Source: CAD feature listing. Evaluate the final solid. Frame: model axes, mm. Give positions to 0.01 mm unless a question says otherwise; leave off trailing zeros. Loops run counter-clockwise (first coordinate to the right, second up) from the corner with the lowest first, then second, coordinate; pieces in that order, holes last. Notation, with made-up numbers: M 2.25,-37.75 L 36.25,-37.75 A21 cw 36.25,-14.75 Z; hole C 52.5,36 d10. An arc over 180 degrees is marked long. Write item = value, one per line.
from build123d import *

# Parameters (mm, degrees)
SKETCH1_4_R         = 3
SKETCH1_4_W         = 5.2
SKETCH1_4_H         = 20.6
BOSS_EXTRUDE2_DEPTH = 4
SKETCH1_5_R         = 3
SKETCH1_5_R_2       = 1
BOSS_EXTRUDE3_DEPTH = 2


with BuildPart() as part:
    # Sketch1_4 → Boss-Extrude2 (new body)
    with BuildSketch(Plane(origin=(0, 0, 0), x_dir=(1, 0, 0), z_dir=(0, 1, 0))):
        Polygon((-61.058774723, -67.225766481), (-46.058774723, -67.225766481), (-46.058774723, -57.925766481), (-16.058774723, -57.925766481), (-16.058774723, -47.925766481), (-46.058065355, -47.925766481), (-46.058065355, -38.625766481), (-46.058774723, 52.774233519), (-46.058774723, 62.074233519), (-16.058774723, 62.074233519), (-16.058774723, 72.074233519), (-46.058065355, 72.074233519), (-46.058065355, 81.374233519), (-61.058065355, 81.374233519), (-61.058065355, 72.074233519), (-111.058065355, 72.074233519), (-111.058065355, 62.074233519), (-61.058774723, 62.074233519), (-61.058774723, 52.774233519), (-61.058065355, -38.625766481), (-61.058065355, -47.925766481), (-111.058065355, -47.925766481), (-111.058065355, -57.925766481), (-61.058774723, -57.925766481), align=None)
        with Locations((-96.731187499, 67.074233519)):
            Circle(SKETCH1_4_R, mode=Mode.SUBTRACT)
        with Locations((-23.608327945, 67.074233519)):
            Circle(SKETCH1_4_R, mode=Mode.SUBTRACT)
        with Locations((-96.731187499, -52.925766481)):
            Circle(SKETCH1_4_R, mode=Mode.SUBTRACT)
        with Locations((-23.608327945, -52.925766481)):
            Circle(SKETCH1_4_R, mode=Mode.SUBTRACT)
        with Locations((-53.558065355, -52.925766481)):
            Rectangle(SKETCH1_4_W, SKETCH1_4_H, mode=Mode.SUBTRACT)
        with Locations((-53.558065355, 67.074233519)):
            Rectangle(SKETCH1_4_W, SKETCH1_4_H, mode=Mode.SUBTRACT)
    extrude(amount=BOSS_EXTRUDE2_DEPTH)

    # Sketch1_5 → Boss-Extrude3 (add)
    with BuildSketch(Plane(origin=(0, 0, 0), x_dir=(1, 0, 0), z_dir=(0, 1, 0))):
        Polygon((-61.058774723, -57.925766481), (-61.058774723, -67.225766481), (-46.058774723, -67.225766481), (-46.058774723, -57.925766481), (-16.058774723, -57.925766481), (-16.058774723, -47.925766481), (-46.058065355, -47.925766481), (-46.058065355, -38.625766481), (-46.058774723, 52.774233519), (-46.058774723, 62.074233519), (-16.058774723, 62.074233519), (-16.058774723, 72.074233519), (-46.058065355, 72.074233519), (-46.058065355, 81.374233519), (-61.058065355, 81.374233519), (-61.058065355, 72.074233519), (-111.058065355, 72.074233519), (-111.058065355, 62.074233519), (-61.058774723, 62.074233519), (-61.058774723, 52.774233519), (-61.058065355, -38.625766481), (-61.058065355, -47.925766481), (-111.058065355, -47.925766481), (-111.058065355, -57.925766481), align=None)
        with Locations((-96.731187499, -52.925766481)):
            Circle(SKETCH1_5_R, mode=Mode.SUBTRACT)
        with Locations((-23.608327945, -52.925766481)):
            Circle(SKETCH1_5_R, mode=Mode.SUBTRACT)
        with Locations((-23.608327945, 67.074233519)):
            Circle(SKETCH1_5_R, mode=Mode.SUBTRACT)
        with Locations((-96.731187499, 67.074233519)):
            Circle(SKETCH1_5_R, mode=Mode.SUBTRACT)
        with Locations((-53.558065355, -58.925766481)):
            Circle(SKETCH1_5_R_2, mode=Mode.SUBTRACT)
        with Locations((-53.558065355, -46.925766481)):
            Circle(SKETCH1_5_R_2, mode=Mode.SUBTRACT)
        with Locations((-53.558065355, 61.074233519)):
            Circle(SKETCH1_5_R_2, mode=Mode.SUBTRACT)
        with Locations((-53.558065355, 73.074233519)):
            Circle(SKETCH1_5_R_2, mode=Mode.SUBTRACT)
    extrude(amount=-BOSS_EXTRUDE3_DEPTH)


solid = part.part
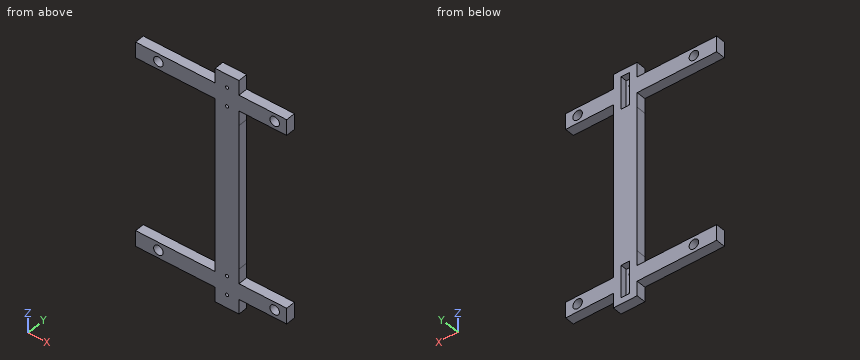
1. Cut plane A-A, the plane x = -104.5. Return the cut outline in (y, z), then the cut area to 3 significant figures.
Derived:
outline = M -2,-72.07 L 4,-72.07 L 4,-62.07 L -2,-62.07 Z; M -2,47.93 L 4,47.93 L 4,57.93 L -2,57.93 Z
area = 120 mm²
2. Cut plane C-C, the plane z = -24.5. Return the cut outline in (x, y).
Derived:
outline = M -61.06,-2 L -46.06,-2 L -46.06,4 L -61.06,4 Z
3. First-contact query: pin 1 Ø3 at (x, z) = (-53.56, 46.93) entering from +Y; pin 2 Ø3 at (y, z) = (0.5, -57) entering from -X; pin 3 Ø1 at (x, y) = (-78.5, 1.5) entering from -Z. Flat tips, straight axial feed; report the tip coordinate or a pass-through.
Derived:
pin_1 = 0
pin_2 = -61.06
pin_3 = -72.07
4. Material intervals for probe 1 along Z at (x, y) = (-82.5, 1.2); probe 2 along Z at (x, y) = (-51, 2.65); probe 3 along X at (y, z) = (-1.4, 55), sorted ascending. Write a range as from..to.
Derived:
probe_1 = -72.07..-62.07, 47.93..57.93
probe_2 = -81.37..-77.37, -56.77..42.63, 63.23..67.23
probe_3 = -111.06..-98.9, -94.56..-25.78, -21.44..-16.06
5. Cut plane B-B, the plane y = 3.1. Count the separate pieces of the cut face and the enclosed holes in it, then the cut area to 3 significant figures.
Derived:
separate_pieces = 1
enclosed_holes = 6
area = 3,500 mm²
